from build123d import *

# Parameters (mm, degrees)
F0_W     = 50
F0_H     = 100
F1_DEPTH = 50
F2_SIZE  = 15
F4_D     = 12
F4_DEPTH = 25
F4_TIP   = 3.6051637142
F5_R     = 5


with BuildPart() as f1:
    # F0 (on Top) → F1 (new body)
    with BuildSketch(Plane.XY):
        with Locations((25, 50)):
            Rectangle(F0_W, F0_H)
    extrude(amount=F1_DEPTH)

    # F2
    f2_edges = [f1.edges().sort_by_distance(p)[0] for p in [
        (50, 50, 50),
    ]]
    chamfer(f2_edges, length=F2_SIZE)

    # F4
    with Locations(Plane(origin=(42.5, 0, 42.5), x_dir=(0, 1, 0), z_dir=(0.7071067812, 0, 0.7071067812))):
        with Locations((25, 0), (75, 0)):
            Hole(F4_D / 2, depth=F4_DEPTH)
            with Locations((0, 0, -(F4_DEPTH + F4_TIP / 2))):  # 118° drill point
                Cone(0, F4_D / 2, F4_TIP, mode=Mode.SUBTRACT)

    # F5
    f5_edges = [f1.edges().sort_by_distance(p)[0] for p in [
        (25, 100, 0),
        (25, 0, 0),
    ]]
    fillet(f5_edges, radius=F5_R)


solid = f1.part
Verification items for the finished model (mm, model axes). A direction names the side the tool comes from. Coordinates: 2 decimals unless noted, no trailing zeros. Order: outer loops, then holes, each group sorted by start corner. A loop starts at its lowest first (then second) coordinate and runs counter-clockwise, first axis right, second up. Notation, with made-up numbers: M -35,24 L -4,24 A23 ccw -4,40 Z; hole C -20,52 d4. An arc over 180 degrees is marked long. One line per item, written item: value. Start each with the question number.
Item 1: Access from +Z, -Z, +X, -X, +Y, -Y to the whole of each face (thin tool, end or side, straight path). Record for faces 5 (the flat face through (42, 49, 43)), 6 (the conical face through (22.095, 25.56, 23.337)).
Item 2: Gauge pin test, flat end, axial feed: pin 1 (2 mm diameter, centred on x = 44, y = 31.5, fed in from +Z). Record the tip position at first contact, or that the pin passes through.
Item 3: Scan lines: probe 1 along X at (y, z) = (70.5, 34.5); probe 2 along X at (y, z) = (80, 26); probe 3 along Z at (x, y) = (32, 71). Record each from-to range of solid material in increasing order.
Item 4: Sectioned sample at B-B (x = 32). Count the separate pieces of the cut face and the enclosed holes in it, then the cut area to 3 significant figures.
Item 5: Mould release check, pull along Z, two halves, no side actions. Record for faces 1 (the conical face through (22.49, 75.99, 22.94)), 2 (the cylindrical face through (25, 98, 1)), 3 (the cylindrical face through (33.351, 80.994, 33.724)), 4 (the flat face through (17, 51, 50)): released by +Z, released by -Z, zero draft, split by the parting line, or undercut.
Item 6: Sectioned sample at A-A (y = 32). Enter the section's corners in (x, z), then the cut area to 3 significant figures.
Conclusion:
1. face 5: +Z, +X, +Y, -Y
1. face 6: none
2. pin 1: stops at z = 42
3. probe 1: x = 0 to 28.89, 40.11 to 50
3. probe 2: x = 0 to 23.13, 30.69 to 50
3. probe 3: z = 0 to 25.68, 38.32 to 50
4. separate pieces: 1
4. enclosed holes: 2
4. area: 4,670 mm^2
5. face 1: undercut
5. face 2: released by -Z
5. face 3: undercut
5. face 4: released by +Z
6. outline: M 0,0 L 50,0 L 50,35 L 35,50 L 0,50 Z
6. area: 2,390 mm^2
